Here's the drawing with two shaded views (mm, measured from the low corner). I have some questions. Coordinates: 2 decimals unless noted, no trailing zeros. Loops run counter-clockwise (first coordinate to the right, second up) from the corner with the lowest first, then second, coordinate; pieces in that order, holes last. Notation, with made-up numbers: M -12.75,1.5 L 45.25,1.5 A37 ccw 45.25,39.5 Z; hole C 75.5,44.25 d5. An arc over 180 degrees is marked long. Return JSON: item names as keys, results as strings. Group by question number.
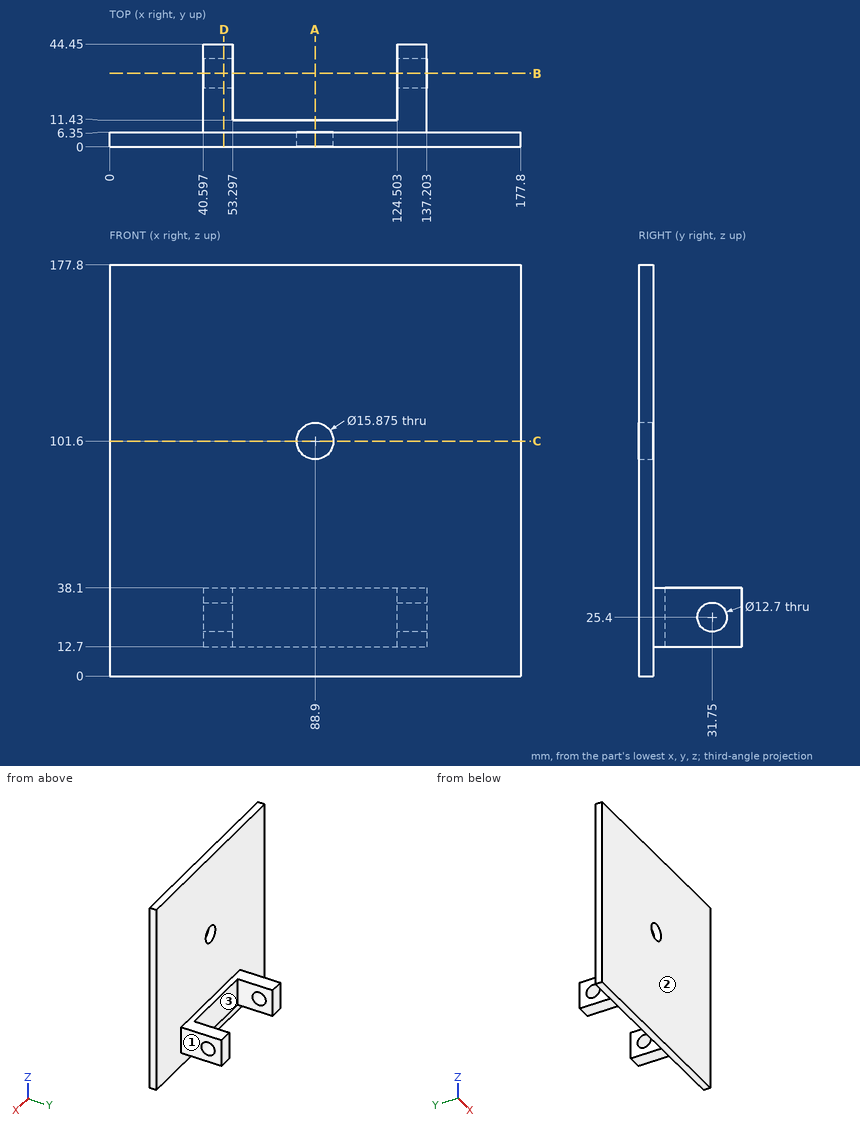
(1) Will these pins go through, and if not, where does the flat tip stop? P1, Ø12.5, axis at x = 90, z = 28.5, coming from the +Y side; P2, Ø14.5, axis at y = 31.75, z = 25.4, coming from the +X side; P3, Ø1, axis at x = 145.5, z = 67.5, coming from the +Y side.
(2) Imagine slicing it at D-D, the plane x = 49.5. Write out the boundary of the cut face in (y, z).
(3) We'd pull the mould along X, two halves only. Please class the marked faces 1, 2 and 3: +X half, -X half, draft (parallel to the pull), parting line (faces both ways), or undercut.
(4) Imagine slicing it at B-B, the plane y = 31.75. Write out the boundary of the cut face in (x, z).
(5) Imagine slicing it at C-C, the plane z = 101.6. Write out the boundary of the cut face in (x, y).
(6) If I drill on L1, parallel to Y at x = 46.5, z = 25.4; L2, parallel to X at y = 38.5, z = 21; L3, parallel to Y at x = 50, z = 149, over which ranges is the centre line in solid material (lowest first)? Write a range as [from, to].
(7) Imagine slicing it at A-A, the plane x = 88.9. Write out the boundary of the cut face in (y, z), then the cut area to 3 significant figures.
Checks:
{
 "1": {"P1": "y = 11.43", "P2": "x = 137.2", "P3": "y = 6.35"},
 "2": {"outline": "M 0,0 L 6.35,0 L 6.35,12.7 L 44.45,12.7 L 44.45,38.1 L 6.35,38.1 L 6.35,177.8 L 0,177.8 Z; hole C 31.75,25.4 d12.7"},
 "3": {"face 1": "+X half", "face 2": "draft", "face 3": "undercut"},
 "4": {"outline": "M 40.6,12.7 L 53.3,12.7 L 53.3,19.05 L 40.6,19.05 Z; M 40.6,31.75 L 53.3,31.75 L 53.3,38.1 L 40.6,38.1 Z; M 124.5,12.7 L 137.2,12.7 L 137.2,19.05 L 124.5,19.05 Z; M 124.5,31.75 L 137.2,31.75 L 137.2,38.1 L 124.5,38.1 Z"},
 "5": {"outline": "M 0,0 L 80.96,0 L 80.96,6.35 L 0,6.35 Z; M 96.84,0 L 177.8,0 L 177.8,6.35 L 96.84,6.35 Z"},
 "6": {"L1": "[0, 25.4], [38.1, 44.45]", "L2": "[40.6, 53.3], [124.5, 137.2]", "L3": "[0, 6.35]"},
 "7": {"outline": "M 0,0 L 6.35,0 L 6.35,12.7 L 11.43,12.7 L 11.43,38.1 L 6.35,38.1 L 6.35,93.66 L 0,93.66 Z; M 0,109.54 L 6.35,109.54 L 6.35,177.8 L 0,177.8 Z", "area": "1,160 mm²"}
}
